Geometry check sheet. Reference: the model listing, model coordinates, mm. A direction names the side the tool comes from. Round coordinates to 2 decimals unless told otherwise and drop trailing zeros. Write each loop counter-clockwise with the first axis right and the second up, starting at its lowest first coordinate (ties: lowest second). Pieces come first, ordered by that corner, then holes. Notation, with made-up numbers: (79, -9) -> (135, -9) arc R22 cw to (135, 16) -> close; hole circle Ø7 at (-35.75, 52). An arc over 180 degrees is marked (long way). Return JSON: item names as keys, results as strings. Group by question number.
Solid Edge part; units mm, degrees
sketch "Sketch1" plane through (0, 0, 0) normal (0, 0, 1) x (1, 0, 0)
  line L0 (0, 25) -> (7.0711, 17.9289)
  line L1 (7.0711, 17.9289) -> (11.3945, 22.2523)
  arc A0 (11.3945, 22.2523) -> (11.3945, -22.2523) centre (0, 0) cw
  line L2 (7.0711, -17.9289) -> (11.3945, -22.2523)
  line L3 (0, -25) -> (7.0711, -17.9289)
  arc A1 (0, 25) -> (0, -25) centre (0, 0) ccw
extrude "Protrusion1" add sketch "Sketch1" along normal mid plane 11
sketch "Sketch2" plane through (0, 0, 5.5) normal (0, 0, 1) x (0.7071, 0.7071, 0)
  circle A0 centre (0, 0) radius 25
  line L0 (-2.6777, -19.8199) -> (-2.6777, -12.6777)
  line L1 (-2.6777, -12.6777) -> (-15.4686, -12.6777)
  arc A1 (12.6777, 15.4686) -> (-15.4686, -12.6777) centre (0, 0) ccw
  line L2 (12.6777, 15.4686) -> (12.6777, 2.6777)
  line L3 (12.6777, 2.6777) -> (19.8199, 2.6777)
  arc A2 (-2.6777, -19.8199) -> (19.8199, 2.6777) centre (0, 0) ccw
extrude "ExtrudedProtrusion_2" add sketch "Sketch2" along normal blind 10
fillet "Round_1" radius 3 6 edges at (7.0711, -10.8579, 10.5) (12.1214, -15.9082, 10.5) (-1.9735, -19.9024, 10.5) (7.0711, 10.8579, 10.5) (12.1214, 15.9082, 10.5) (-1.9735, 19.9024, 10.5)
sketch "Sketch3" plane through (0, 0, 15.5) normal (0, 0, 1) x (-1, 0, 0)
  circle A0 centre (0, 0) radius 25
  circle A1 centre (0, 0) radius 20
extrude "ExtrudedProtrusion_3" add sketch "Sketch3" along normal blind 70
mirror "Mirror1" about plane through (0, 0, 0) normal (0, 0, 1) of "ExtrudedProtrusion_2", "Round_1", "ExtrudedProtrusion_3"
properties material "PVC"
1) Tool access check on faces 1 (the face through (7.1, -12.1, 10.6)), 2 (the face through (6, -22, 5.5)), 3 (the face through (6, 22, 5.5)), 4 (the face through (11, 17, -85.5)), 5 (the face through (7, -12.1, -10.6)). Record the directions out of +Z, -Z, +X, -X, +Y, -Y that give a thin tool (end or side, any length) a straight path to the whole face; none if there is none.
2) Mould release check, pull along X, two halves, no side actions. Record for faces 6 (the face through (-11, 17, 85.5)), 7 (the face through (5, -16, 15.5)): +X half, -X half, draft (parallel to the pull), parting line (faces both ways), or undercut.
3) Sectioned sample at A-A on y = -7. Enter the section's corners in (x, z) (3 decimals).
4) Material ranges on probe 1 along Y at (x, z) = (0, -50.5); probe 2 along Z at (x, y) = (6, -23), recorded low to high. Write a range as [from, to].
5) Sectioned sample at C-C on x = 16. Enter the section's corners in (y, z).
6) Sectioned sample at B-B on z = 20.5. Enter the section's corners in (x, y), and give its area (3 significant figures).
7) Go/stop test with flat-tipped pins: P1, Ø8, axis at x = 1.5, y = 3.5, coming from the -Z side; P2, Ø12, axis at y = -19, z = -61.5, coming from the +X side; P3, Ø0.6, axis at x = 7, y = 12, coming from the -Z side. Record where each tip stops, or that it passes through.
Evaluation:
{
 "1": {"face 1": "+Z", "face 2": "-Y", "face 3": "+Y", "face 4": "-Z, +X, -X, +Y, -Y", "face 5": "-Z"},
 "2": {"face 6": "draft", "face 7": "undercut"},
 "3": {"outline": "(-24, -85.5) -> (-18.735, -85.5) -> (-18.735, -5.5) -> (18.735, -5.5) -> (18.735, -85.5) -> (24, -85.5) -> (24, 85.5) -> (18.735, 85.5) -> (18.735, 5.5) -> (-18.735, 5.5) -> (-18.735, 85.5) -> (-24, 85.5) -> close"},
 "4": {"probe 1": "y = [-25, -20], [20, 25]", "probe 2": "z = [-85.5, -5.5], [5.5, 85.5]"},
 "5": {"outline": "(-19.21, -85.5) -> (-12, -85.5) -> (-12, -5.5) -> (12, -5.5) -> (12, -85.5) -> (19.21, -85.5) -> (19.21, 85.5) -> (12, 85.5) -> (12, 5.5) -> (-12, 5.5) -> (-12, 85.5) -> (-19.21, 85.5) -> close"},
 "6": {"outline": "circle Ø50 at (0, 0); hole circle Ø40 at (0, 0)", "area": "707 mm2"},
 "7": {"P1": "stops at z = -5.5", "P2": "stops at x = 21.35", "P3": "stops at z = -15.5"}
}
